Geometry: final body of the model. Coordinates: model frame, mm. Face numbers are marked on the shaded views. A direction names the side the tool comes from. Round coordinates to 2 decimals unless told otherwise and drop trailing zeros. Loops run counter-clockwise (first coordinate to the right, second up) from the corner with the lowest first, then second, coordinate; pieces in that order, holes last. Notation, with made-up numbers: (51.25, 74.5) - (97.25, 74.5) arc R18 cw to (97.25, 84.5) - close; hole circle Ø4 at (45.25, -27.75). An arc over 180 degrees is marked (long way). Answer as CSV lines item,"result".
from build123d import *

# Parameters (mm, degrees)
CROQUIS1_R              = 11.05
CROQUIS1_R_2            = 2.5
SALIENTE_EXTRUIR1_DEPTH = 10
CROQUIS2_R              = 13
CROQUIS2_R_2            = 9.5
SALIENTE_EXTRUIR2_DEPTH = 3


with BuildPart() as part:
    # Croquis1 → Saliente-Extruir1 (new body)
    with BuildSketch(Plane.XY):
        with BuildLine():
            Line((-57.878391193, 30.074329664), (-57.878391193, 0.074329664))
            ThreePointArc((-57.878391193, 0.074329664), (-52.378391193, -5.425670336), (-46.878391193, 0.074329664))
            Line((-46.878391193, 0.074329664), (-27.878391193, 0.074329664))
            ThreePointArc((-27.878391193, 0.074329664), (-22.378391193, -5.425670336), (-16.878391193, 0.074329664))
            Line((-16.878391193, 0.074329664), (-16.878391193, 30.074329664))
            ThreePointArc((-16.878391193, 30.074329664), (-22.378391193, 35.574329664), (-27.878391193, 30.074329664))
            Line((-27.878391193, 30.074329664), (-46.878391193, 30.074329664))
            ThreePointArc((-46.878391193, 30.074329664), (-52.378391193, 35.574329664), (-57.878391193, 30.074329664))
        make_face()
        with Locations((-37.378391193, 15.074329664)):
            Circle(CROQUIS1_R, mode=Mode.SUBTRACT)
        with Locations((-22.378391193, 0.074329664)):
            Circle(CROQUIS1_R_2, mode=Mode.SUBTRACT)
        with Locations((-52.378391193, 0.074329664)):
            Circle(CROQUIS1_R_2, mode=Mode.SUBTRACT)
        with Locations((-52.378391193, 30.074329664)):
            Circle(CROQUIS1_R_2, mode=Mode.SUBTRACT)
        with Locations((-22.378391193, 30.074329664)):
            Circle(CROQUIS1_R_2, mode=Mode.SUBTRACT)
    extrude(amount=SALIENTE_EXTRUIR1_DEPTH)

    # Croquis2 → Saliente-Extruir2 (add)
    with BuildSketch(Plane.XY.offset(10)):
        with Locations((-37.378391193, 15.074329664)):
            Circle(CROQUIS2_R)
        with Locations((-37.378391193, 15.074329664)):
            Circle(CROQUIS2_R_2, mode=Mode.SUBTRACT)
    extrude(amount=-SALIENTE_EXTRUIR2_DEPTH)


solid = part.part
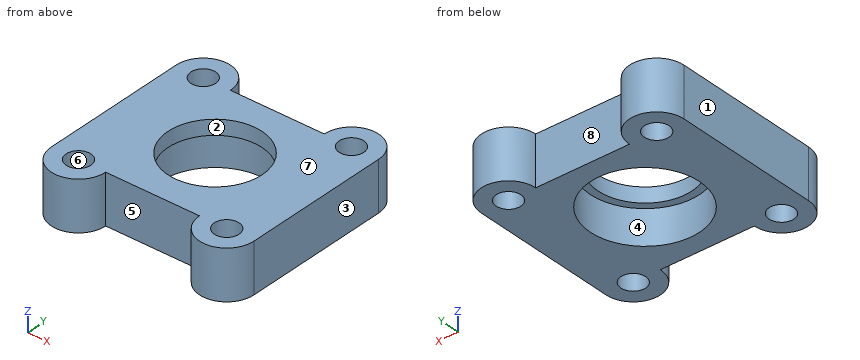
(1) Section D-D (y = 9.5). Output: boundary loops of the cut face in (x, z).
Findings below:
outline,"(-57.88, 0) - (-46.92, 0) - (-46.92, 7) - (-45.07, 7) - (-45.07, 10) - (-57.88, 10) - close; (-29.69, 7) - (-27.84, 7) - (-27.84, 0) - (-16.88, 0) - (-16.88, 10) - (-29.69, 10) - close"
(2) Section B-B (y = 32). Output: boundary loops of the cut face in (x, z).
Findings below:
outline,"(-57.53, 0) - (-53.97, 0) - (-53.97, 10) - (-57.53, 10) - close; (-50.78, 0) - (-47.23, 0) - (-47.23, 10) - (-50.78, 10) - close; (-27.53, 0) - (-23.97, 0) - (-23.97, 10) - (-27.53, 10) - close; (-20.78, 0) - (-17.23, 0) - (-17.23, 10) - (-20.78, 10) - close"
(3) Pin query (flat end, axial travel): P1, Ø5, axis at x = -40.5, z = 6.5, coming from the +Y side; P2, Ø2, axis at x = -45.5, z = 8.5, coming from the -Y side. Return the tip coordinate at first contact, or that it passes through.
Findings below:
P1,"y = 30.07"
P2,"y = 0.07"
(4) Access query for the marked faces 4, 5, 6, 7 and 8. Directions: +Z, -Z, +X, -X, +Y, -Y. A direction counts if a zero-diameter tool reaches every point of the face in a straight line with its end or side. Return the directions, or none.
Findings below:
face 4,"-Z"
face 5,"+Z, -Z, -Y"
face 6,"+Z, -Z"
face 7,"+Z, +X, -X, +Y, -Y"
face 8,"+Z, -Z, +Y"
(5) Section C-C (z = 3.25). Output: boundary loops of the cut face in (x, y).
Findings below:
outline,"(-57.88, 0.07) arc R5.5 ccw to (-46.88, 0.07) - (-27.88, 0.07) arc R5.5 ccw to (-16.88, 0.07) - (-16.88, 30.07) arc R5.5 ccw to (-27.88, 30.07) - (-46.88, 30.07) arc R5.5 ccw to (-57.88, 30.07) - close; hole circle Ø5 at (-52.38, 0.07); hole circle Ø5 at (-52.38, 30.07); hole circle Ø22.1 at (-37.38, 15.07); hole circle Ø5 at (-22.38, 0.07); hole circle Ø5 at (-22.38, 30.07)"
(6) Material intervals for line 1 along Y through (x, z) = (-37, 2.5); line 2 along Y through (x, z) = (-21.5, 3.25); line 3 along Y through (x, z) = (-20.5, 5.75), sorted ascending.
Findings below:
line 1,"0.07 to 4.03, 26.12 to 30.07"
line 2,"-5.36 to -2.27, 2.41 to 27.73, 32.41 to 35.5"
line 3,"-5.09 to -1.58, 1.72 to 28.42, 31.72 to 35.24"
(7) Section A-A (x = -28.5). Output: boundary loops of the cut face in (y, z).
Findings below:
outline,"(0.07, 0) - (8.5, 0) - (8.5, 7) - (11.69, 7) - (11.69, 10) - (0.07, 10) - close; (18.45, 7) - (21.65, 7) - (21.65, 0) - (30.07, 0) - (30.07, 10) - (18.45, 10) - close"
(8) Draft query along X for the marked faces 1, 2 and 3. Return one class per face: pulls with the +X half, pulls with the -X half, needs draft (parallel to the pull), parting line crosses it, or undercut.
Findings below:
face 1,"pulls with the -X half"
face 2,"undercut"
face 3,"pulls with the +X half"
